The model under review builds one solid part; all positions refer to its coordinate system, in mm. Face numbers are marked on the shaded views. A direction names the side the tool comes from. Give positions to 0.01 mm unless a question says otherwise; leave off trailing zeros. Loops run counter-clockwise (first coordinate to the right, second up) from the corner with the lowest first, then second, coordinate; pieces in that order, holes last. Notation, with made-up numbers: M 86.5,-5.75 L 91.5,-5.75 A33 cw 91.5,29.25 Z; hole C -30.5,-24 d7. An arc over 180 degrees is marked long. Return JSON: item names as keys, results as strings.
```python
from build123d import *

# Parameters (mm, degrees)
BOSS_EXTRUDE1_DEPTH = 50
SKETCH3_R           = 1.6
CUT_EXTRUDE1_DEPTH  = 50
SKETCH4_R           = 5
CUT_EXTRUDE2_DEPTH  = 50
FILLET1_R           = 10
FILLET2_R           = 6
FILLET3_R           = 10


with BuildPart() as part:
    # Sketch2 → Boss-Extrude1 (new body)
    with BuildSketch(Plane.XY):
        Polygon((0, 0), (-95, 0), (-95, -28), (-91, -28), (-91, -4), (-4, -4), (-4, -60), (0, -60), align=None)
    extrude(amount=BOSS_EXTRUDE1_DEPTH)

    # Sketch3 → Cut-Extrude1 (cut)
    with BuildSketch(Plane.ZY.offset(95)):
        with Locations((12.5, -20)):
            Circle(SKETCH3_R)
        with Locations((37.5, -20)):
            Circle(SKETCH3_R)
    extrude(amount=-CUT_EXTRUDE1_DEPTH, mode=Mode.SUBTRACT)

    # Sketch4 → Cut-Extrude2 (cut)
    with BuildSketch(Plane(origin=(0, 0, 0), x_dir=(0, 0, -1), z_dir=(1, 0, 0))):
        with Locations((-14.8, -42.25)):
            Circle(SKETCH4_R)
    extrude(amount=-CUT_EXTRUDE2_DEPTH, mode=Mode.SUBTRACT)

    # Fillet1
    fillet1_edges = [part.edges().sort_by_distance(p)[0] for p in [
        (-95, 0, 25),
        (0, 0, 25),
    ]]
    fillet(fillet1_edges, radius=FILLET1_R)

    # Fillet2
    fillet2_edges = [part.edges().sort_by_distance(p)[0] for p in [
        (-4, -4, 25),
        (-91, -4, 25),
    ]]
    fillet(fillet2_edges, radius=FILLET2_R)

    # Fillet3
    fillet3_edges = [part.edges().sort_by_distance(p)[0] for p in [
        (-93, -28, 0),
        (-93, -28, 50),
        (-2, -60, 50),
        (-2, -60, 0),
    ]]
    fillet(fillet3_edges, radius=FILLET3_R)


solid = part.part
```
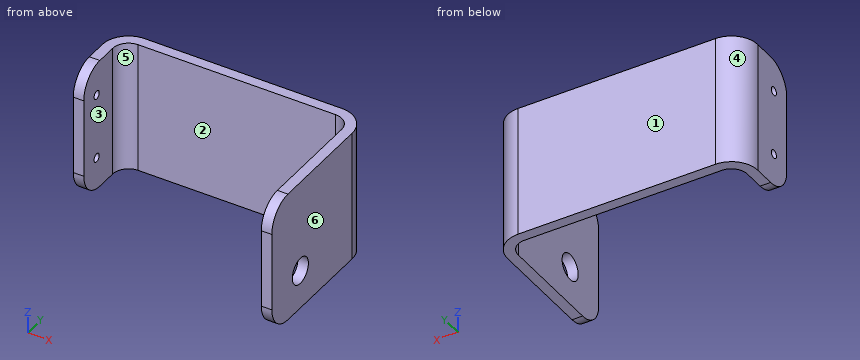
1) Tool access review of the marked faces 5 and 6: name each direction out of +Z, -Z, +X, -X, +Y, -Y from which nothing blocks a thin tool from reaching the whole face with its end or side.
From the geometry:
{"face 5": "+Z, -Z, -Y", "face 6": "+Z, -Z, +X, +Y, -Y"}
2) Wall thickness on L1, parallel to X at y = -13, z = 5.5; L2, parallel to Y at x = -38, z = 5.5: over which ranges is each line inside the solid? List them lowest first. Write a range as from..to.
From the geometry:
{"L1": "-95..-91, -4..0", "L2": "-4..0"}
3) Consider section A-A on y = -42.25. Write out the cut boundary in (x, z), then the cut area to 3 significant figures.
From the geometry:
{"outline": "M -4,0 L 0,0 L 0,9.8 L -4,9.8 Z; M -4,19.8 L 0,19.8 L 0,50 L -4,50 Z", "area": "160 mm²"}
4) Consider section C-C on y = -20. Write out the cut boundary in (x, z).
From the geometry:
{"outline": "M -95,0.2 L -91,0.2 L -91,10.9 L -95,10.9 Z; M -95,14.1 L -91,14.1 L -91,35.9 L -95,35.9 Z; M -95,39.1 L -91,39.1 L -91,49.8 L -95,49.8 Z; M -4,0 L 0,0 L 0,50 L -4,50 Z"}
5) Insertion check: pin 1 (4.5 mm diameter, centred on x = -93, z = 26, fed in from -Y); pin 2 (5 mm diameter, centred on x = -15.5, z = 20, fed in from -Y); pin 3 (4 mm diameter, centred on y = -35.5, z = 9.5, fed in from -X). Each pin has a flat end and moves straight along its axis. Give the tip position at first contact, or say it passes through.
From the geometry:
{"pin 1": "y = -28", "pin 2": "y = -4", "pin 3": "x = -4"}
6) Consider section B-B on z = 37.5. Write out the cut boundary in (x, y).
From the geometry:
{"outline": "M -95,-28 L -91,-28 L -91,-21.6 L -95,-21.6 Z; M -95,-18.4 L -91,-18.4 L -91,-10 A6 cw -85,-4 L -10,-4 A6 cw -4,-10 L -4,-60 L 0,-60 L 0,-10 A10 ccw -10,0 L -85,0 A10 ccw -95,-10 Z"}
7) Consider section D-D on z = 12.5. Write out the cut boundary in (x, y).
From the geometry:
{"outline": "M -95,-28 L -91,-28 L -91,-21.6 L -95,-21.6 Z; M -95,-18.4 L -91,-18.4 L -91,-10 A6 cw -85,-4 L -10,-4 A6 cw -4,-10 L -4,-37.81 L 0,-37.81 L 0,-10 A10 ccw -10,0 L -85,0 A10 ccw -95,-10 Z; M -4,-60 L 0,-60 L 0,-46.69 L -4,-46.69 Z"}
8) The part is to be moulded in two halves that separate along X. For the marked faces 1, 2, 3 and 4, say which applies: released by +X, released by -X, zero draft, split by the parting line, or undercut.
From the geometry:
{"face 1": "zero draft", "face 2": "undercut", "face 3": "undercut", "face 4": "released by -X"}
